Design review of the part built by this model. Coordinates are the model's own, in mm. A direction names the side the tool comes from. Coordinates: 2 decimals unless noted, no trailing zeros. Loops run counter-clockwise (first coordinate to the right, second up) from the corner with the lowest first, then second, coordinate; pieces in that order, holes last. Notation, with made-up numbers: (41.25, 12.5) -> (55.25, 12.5) arc R13 cw to (55.25, 30.5) -> close; hole circle Ø10 at (43.5, 16). An arc over 180 degrees is marked (long way). Use a Markdown table: item, result. Add a question column.
Q1. Take a section at A-A on x = 0. Write out the cut boundary in (y, z), plus the area to 3 significant figures.
Q2. Take a section at B-B on y = -6.25. Write out the cut boundary in (x, z).
Q3. Clearance check with flat-ended pins moving along their axes: pin 1 Ø13.5 at (x, z) = (0, 0) entering from -Y; pin 2 Ø3 at (x, y) = (9, -5) entering from -Z; pin 3 Ø3 at (x, y) = (-6.5, -7) entering from -Z; pin 4 Ø3 at (x, y) = (8.5, -6) entering from +Z. State where each tip first meets the part, or that it passes through.
Q4. Draft analysis for pull direction X (two halves, no side actions). For faces 1 (the face through (0, -10, 185)), 2 (the face through (-0.651, -4.93, 129.957)), 3 (the face through (15, -5, 234)), 4 (the face through (-0.16, -4.93, 482.5)), state which applies: pulls with the +X half, pulls with the -X half, needs draft (parallel to the pull), parting line crosses it, or undercut.
Q5. For faces 5 (the face through (-15, -5, 241)), 6 (the face through (-7.5, -5, 399)), list the 3-axis set-ups (+Z, -Z, +X, -X, +Y, -Y) from which the entire face can be reached by the end or side of a thin tool; tool diameter is ignored.
Q6. For probe 1 along Z at (x, y) = (0, -4); probe 2 along Z at (x, y) = (-4.5, -3.5); probe 3 along X at (y, z) = (-7.75, 406), list the stretches that pass through material, from the lowest coordinate up.
from build123d import *

# Parameters (mm, degrees)
F0_R     = 7.5
F0_R_2   = 5
F1_DEPTH = 10


with BuildPart() as f1:
    # F0 (on Front) → F1 (new body)
    with BuildSketch(Plane.XZ):
        with BuildLine():
            Line((-15, 475), (-15, 0))
            ThreePointArc((-15, 0), (0, -15), (15, 0))
            Line((15, 0), (15, 475))
            ThreePointArc((15, 475), (0, 490), (-15, 475))
        make_face()
        Circle(F0_R, mode=Mode.SUBTRACT)
        with Locations((0, 125)):
            Circle(F0_R_2, mode=Mode.SUBTRACT)
        with BuildLine():
            ThreePointArc((-7.5, 475), (0, 482.5), (7.5, 475))
            Line((7.5, 475), (7.5, 325))
            ThreePointArc((7.5, 325), (0, 317.5), (-7.5, 325))
            Line((-7.5, 325), (-7.5, 475))
        make_face(mode=Mode.SUBTRACT)
    extrude(amount=F1_DEPTH)


solid = f1.part
Answer list:
| question | item | result |
|---|---|---|
| 1 | outline | (-10, -15) -> (0, -15) -> (0, -7.5) -> (-10, -7.5) -> close; (-10, 7.5) -> (0, 7.5) -> (0, 120) -> (-10, 120) -> close; (-10, 130) -> (0, 130) -> (0, 317.5) -> (-10, 317.5) -> close; (-10, 482.5) -> (0, 482.5) -> (0, 490) -> (-10, 490) -> close |
| 1 | area | 3,150 mm² |
| 2 | outline | (-15, 0) arc R15 ccw to (15, 0) -> (15, 475) arc R15 ccw to (-15, 475) -> close; hole circle Ø15 at (0, 0); hole (-7.5, 325) arc R7.5 ccw to (7.5, 325) -> (7.5, 475) arc R7.5 ccw to (-7.5, 475) -> close; hole circle Ø10 at (0, 125) |
| 3 | pin 1 | through |
| 3 | pin 2 | z = -12.99 |
| 3 | pin 3 | z = -14.14 |
| 3 | pin 4 | z = 488.27 |
| 4 | face 1 | needs draft |
| 4 | face 2 | undercut |
| 4 | face 3 | pulls with the +X half |
| 4 | face 4 | undercut |
| 5 | face 5 | +Z, -Z, -X, +Y, -Y |
| 5 | face 6 | +Y, -Y |
| 6 | probe 1 | -15 to -7.5, 7.5 to 120, 130 to 317.5, 482.5 to 490 |
| 6 | probe 2 | -14.31 to -6, 6 to 122.82, 127.18 to 319, 481 to 489.31 |
| 6 | probe 3 | -15 to -7.5, 7.5 to 15 |
